Input: part model. Units: mm. Frame: model coordinates. A direction names the side the tool comes from. Give positions to 0.01 mm unless a question says otherwise; leave off trailing zeros. Loops run counter-clockwise (first coordinate to the right, second up) from the corner with the lowest first, then second, coordinate; pieces in that order, holes last. Notation, with made-up numbers: M -27.75,73 L -22.75,73 A8 cw -22.75,85 Z; hole C 3,21 d10. An arc over 180 degrees is marked long. Use CSV: the item, a comma, the result in double quotes. Start each with the question number.
Q1. Reachability of faces 4 (the flat face through (-4, -298, 440)), 5 (the flat face through (-4, -542.999, -381)) from +Z, -Z, +X, -X, +Y, -Y: full face, straight path, thin tool, end or side. Return the list, or none.
Q2. Pull-direction query (Z, two-part tool) for faces 1 (the flat face through (-24, -605, -25)), 2 (the flat face through (-4, -574, -324)), 3 (the flat face through (-4, -625, -157)); classes: released by +Z, released by -Z, zero draft, split by the parting line, or undercut.
Q3. Pin query (flat end, axial travel): pin 1 (16.5 mm diameter, centred on x = -137, y = -611, fed in from -Z); pin 2 (16.5 mm diameter, centred on x = 24.5, y = -615.5, fed in from -Z); pin 3 (7.5 mm diameter, centred on x = -25, y = -614, fed in from +Z). Return the tip coordinate at first contact, or that it passes through.
Q4. Material intervals for line 1 along Y through (x, z) = (-11.5, -292), sorted ascending.
Q5. Section A-A, the plane x = -245. Output: boundary loops of the cut face in (y, z).
from build123d import *

# Parameters (mm, degrees)
F0_W     = 605
F0_H     = 880
F1_DEPTH = 605
F2_W     = 605
F2_H     = 116
F3_DEPTH = 62.0014
F4_W     = 560
F4_H     = 140
F5_DEPTH = 20
F6_W     = 560
F6_H     = 255
F7_DEPTH = 20
F8_W     = 560
F8_H     = 255
F9_DEPTH = 20
F10_R    = 5.08


with BuildPart() as f1:
    # F0 (on Front) → F1 (new body)
    with BuildSketch(Plane.XZ):
        Rectangle(F0_W, F0_H)
    extrude(amount=F1_DEPTH)

    # F2 (on face) → F3 (cut)
    with BuildSketch(Plane.XZ.offset(605)):
        with Locations((0, -382)):
            Rectangle(F2_W, F2_H)
    extrude(amount=-F3_DEPTH, mode=Mode.SUBTRACT)

    # F4 (on face) → F5 (join)
    with BuildSketch(Plane.XZ.offset(605)):
        with Locations((0, 343)):
            Rectangle(F4_W, F4_H)
    extrude(amount=F5_DEPTH)

    # F6 (on face) → F7 (join)
    with BuildSketch(Plane.XZ.offset(605)):
        with Locations((0, 120.5)):
            Rectangle(F6_W, F6_H)
    extrude(amount=F7_DEPTH)

    # F8 (on face) → F9 (join)
    with BuildSketch(Plane.XZ.offset(605)):
        with Locations((0, -158.5)):
            Rectangle(F8_W, F8_H)
    extrude(amount=F9_DEPTH)

    # F10
    f10_edges = [f1.edges().sort_by_distance(p)[0] for p in [
        (0, -625, 413),
        (-280, -625, 343),
        (0, -625, 273),
        (280, -625, 343),
        (0, -625, 248),
        (280, -625, 120.5),
        (-280, -625, 120.5),
        (0, -625, -7),
        (0, -625, -31),
        (-280, -625, -158.5),
        (0, -625, -286),
        (280, -625, -158.5),
    ]]
    fillet(f10_edges, radius=F10_R)


solid = f1.part
A:
1,face 4,"+Z, +X, -X, +Y, -Y"
1,face 5,"-Z, +X, -X, -Y"
2,face 1,"undercut"
2,face 2,"released by -Z"
2,face 3,"zero draft"
3,pin 1,"z = -324"
3,pin 2,"z = -286"
3,pin 3,"z = 413"
4,line 1,"-605 to 0"
5,outline,"M -625,-280.92 A5.08 ccw -619.92,-286 L -605,-286 L -605,-324 L -543,-324 L -543,-440 L 0,-440 L 0,440 L -605,440 L -605,413 L -619.92,413 A5.08 ccw -625,407.92 L -625,278.08 A5.08 ccw -619.92,273 L -605,273 L -605,248 L -619.92,248 A5.08 ccw -625,242.92 L -625,-1.92 A5.08 ccw -619.92,-7 L -605,-7 L -605,-31 L -619.92,-31 A5.08 ccw -625,-36.08 Z"
